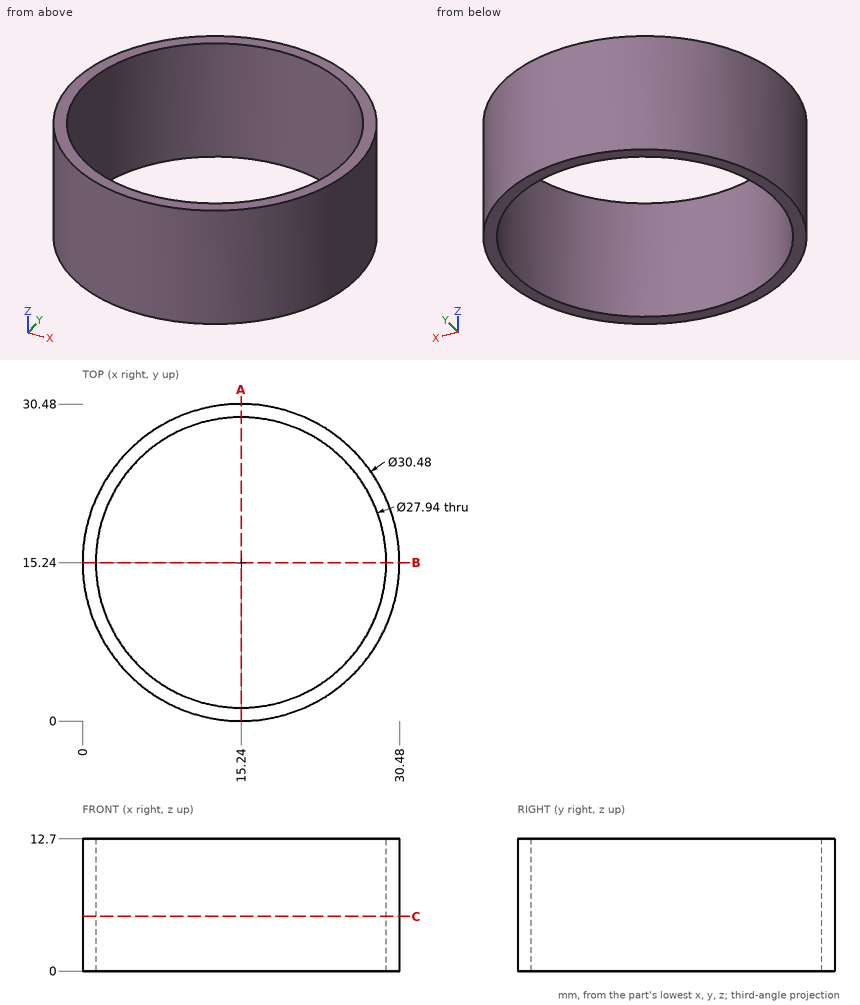
Design review of the part shown in the three views and the two pictorial views. Dimensions are in mm from the part's minimum x, y and z. Give positions to 0.01 mm unless a question says otherwise; leave off trailing zeros. Loops run counter-clockwise (first coordinate to the right, second up) from the corner with the lowest first, then second, coordinate; pieces in that order, holes last. Notation, with made-up numbers: (60, 55) -> (109, 55) arc R33 cw to (109, 90) -> close; hole circle Ø5 at (4, -26.5). An arc over 180 degrees is marked (long way). Answer as a JSON object with one key per item and string values. Group by question number.
Q1. Wall thickness on line 1 along Y through (x, z) = (15, 5.75); line 2 along Y through (x, z) = (3, 1); line 3 along X through (y, z) = (21.5, 12): over which ranges is each line inside the solid? List them lowest first.
Q2. Take a section at A-A (x = 15.24). Write out the cut boundary in (y, z).
Q3. Insertion check: pin 1 (3 mm diameter, centred on y = 23, z = 7.5, fed in from -X); pin 2 (6 mm diameter, centred on y = 12, z = 1.5, fed in from +X); pin 3 (3 mm diameter, centred on x = 9.5, z = 7, fed in from -Y); pin 4 (2 mm diameter, centred on x = 20, y = 25.5, fed in from -Z). Each pin has a flat end and moves straight along its axis. Give the tip position at first contact, or say it passes through.
Q4. Take a section at C-C (z = 5.25). Write out the cut boundary in (x, y), plus the area to 3 significant figures.
Answer below:
{
 "1": {"line 1": "y = 0 to 1.27, 29.21 to 30.48", "line 2": "y = 6.16 to 8.51, 21.97 to 24.32", "line 3": "x = 1.35 to 2.75, 27.73 to 29.13"},
 "2": {"outline": "(0, 0) -> (1.27, 0) -> (1.27, 12.7) -> (0, 12.7) -> close; (29.21, 0) -> (30.48, 0) -> (30.48, 12.7) -> (29.21, 12.7) -> close"},
 "3": {"pin 1": "stops at x = 1.35", "pin 2": "stops at x = 30.48", "pin 3": "stops at y = 0.6", "pin 4": "passes through"},
 "4": {"outline": "circle Ø30.48 at (15.24, 15.24); hole circle Ø27.94 at (15.24, 15.24)", "area": "117 mm2"}
}
